```python
from build123d import *

# Parameters (mm, degrees)
F1_DEPTH  = 4
F3_DEPTH  = 7
F5_DEPTH  = 4
F6_R      = 9
F7_DEPTH  = 4
F8_R      = 9
F9_DEPTH  = 4
F10_R     = 2.5
F11_DEPTH = 1.5
F12_R     = 93.772443
F13_DEPTH = 12.5
F14_R     = 1.5
F15_DEPTH = 11.001
F16_R     = 1.5
F17_DEPTH = 15.001
F18_R     = 2.5
F19_DEPTH = 1.5
F21_DEPTH = 11.001


with BuildPart() as f1:
    # F0 (on Right) → F1 (new body)
    with BuildSketch(Plane.YZ):
        with BuildLine():
            ThreePointArc((37.834946, 8.735705), (19.737718, 6.302024), (1.543294, 7.849729))
            ThreePointArc((1.543294, 7.849729), (-8, 0), (1.543294, -7.849729))
            ThreePointArc((1.543294, -7.849729), (19.737718, -6.302024), (37.834946, -8.735705))
            ThreePointArc((37.834946, -8.735705), (49, 0), (37.834946, 8.735705))
        make_face()
    extrude(amount=F1_DEPTH)

    # F2 (on face) → F3 (join)
    with BuildSketch(Plane.YZ.offset(4)):
        with BuildLine():
            ThreePointArc((13.623219, -6.376131), (25.815239, -6.671862), (37.834946, -8.735705))
            ThreePointArc((37.834946, -8.735705), (49, 0), (37.834946, 8.735705))
            ThreePointArc((37.834946, 8.735705), (19.737718, 6.302024), (1.543294, 7.849729))
            ThreePointArc((1.543294, 7.849729), (0.775296, 7.962344), (0, 8))
            Line((0, 8), (0, 6))
            ThreePointArc((0, 6), (2.468627, 5.468627), (4.5, 3.968627))
            Line((4.5, 3.968627), (13.623219, -6.376131))
        make_face()
    extrude(amount=F3_DEPTH)

    # F4 (on face) → F5 (join)
    with BuildSketch(Plane.YZ.offset(11)):
        with BuildLine():
            ThreePointArc((37.834946, 8.735705), (19.737718, 6.302024), (1.543294, 7.849729))
            ThreePointArc((1.543294, 7.849729), (0.775296, 7.962344), (0, 8))
            ThreePointArc((0, 8), (-7.962344, -0.775296), (1.543294, -7.849729))
            ThreePointArc((1.543294, -7.849729), (7.556447, -6.893156), (13.623219, -6.376131))
            ThreePointArc((13.623219, -6.376131), (25.815239, -6.671862), (37.834946, -8.735705))
            ThreePointArc((37.834946, -8.735705), (49, 0), (37.834946, 8.735705))
        make_face()
    extrude(amount=F5_DEPTH)

    # F6 (on face) → F7 (cut)
    with BuildSketch(Plane.YZ.offset(15)):
        with Locations((40, 0)):
            Circle(F6_R)
    extrude(amount=-F7_DEPTH, mode=Mode.SUBTRACT)

    # F8 (on face) → F9 (cut)
    with BuildSketch(Plane(origin=(0, 0, 0), x_dir=(0, -1, 0), z_dir=(-1, 0, 0))):
        with Locations((-40, 0)):
            Circle(F8_R)
    extrude(amount=-F9_DEPTH, mode=Mode.SUBTRACT)

    # F10 (on face) → F11 (cut)
    with BuildSketch(Plane(origin=(0, 0, 0), x_dir=(0, -1, 0), z_dir=(-1, 0, 0))):
        Circle(F10_R)
    extrude(amount=-F11_DEPTH, mode=Mode.SUBTRACT)

    # F12 (on Top) → F13 (cut, symmetric)
    with BuildSketch(Plane.XY):
        with Locations((-92, 19.68912)):
            Circle(F12_R)
        with Locations((107, 19.68912)):
            Circle(F12_R)
    extrude(amount=F13_DEPTH, both=True, mode=Mode.SUBTRACT)

    # F14 (on face) → F15 (cut, through all)
    with BuildSketch(Plane.YZ.offset(11)):
        with Locations((40, 0)):
            Circle(F14_R)
    extrude(amount=-F15_DEPTH, mode=Mode.SUBTRACT)

    # F16 (on face) → F17 (cut, through all)
    with BuildSketch(Plane.YZ.offset(15)):
        Circle(F16_R)
    extrude(amount=-F17_DEPTH, mode=Mode.SUBTRACT)

    # F18 (on face) → F19 (cut)
    with BuildSketch(Plane.YZ.offset(15)):
        Circle(F18_R)
    extrude(amount=-F19_DEPTH, mode=Mode.SUBTRACT)

    # F20 (on face) → F21 (cut, through all)
    with BuildSketch(Plane.YZ.offset(11)):
        with BuildLine():
            ThreePointArc((40, 7), (46.67877, 2.096194), (44, -5.744563))
            Line((44, -5.744563), (39.357692, -8.977051))
            ThreePointArc((39.357692, -8.977051), (48.994261, -0.321359), (40, 9))
            Line((40, 9), (40, 7))
        make_face()
    extrude(amount=-F21_DEPTH, mode=Mode.SUBTRACT)


solid = f1.part
```
Work out the finished part from the listing and answer in its coordinate system (mm). A direction names the side the tool comes from. Give positions to 0.01 mm unless a question says otherwise; leave off trailing zeros. Loops run counter-clockwise (first coordinate to the right, second up) from the corner with the lowest first, then second, coordinate; pieces in that order, holes last. Notation, with made-up numbers: (55, 33.25) -> (65, 33.25) arc R16 cw to (65, 54.25) -> close; hole circle Ø7 at (-27.75, 77.5). An arc over 180 degrees is marked (long way). One line per question, with ' | ' between items. Start each with the question number.
1) Section A-A, the plane x = 10.5 is taken. Determine the outline of the cut face in (y, z).
2) Section B-B, the plane z = 0 is taken. State how many separate pieces and enclosed holes the cut face has, then the cut area to 3 significant figures.
3) Determine the mould class of faces 1 (the face through (11, 0, -2)), 2 (the face through (9.42, 0.79, 7.96)), 3 (the face through (7.55, 38.5, 0.07)), 4 (the face through (7.5, 2.4, 5.5)) for opening direction Z: +Z half, -Z half, draft (parallel to the pull), parting line (faces both ways), or undercut.
4) Section C-C, the plane y = 24 is taken. Determine the outline of the cut face in (x, z).
5) For faces 5 (the face through (11, 37, 0)), 6 (the face through (0.74, -2.385, 0.751)), 7 (the face through (7.451, 8.998, -1.131)), 8 (the face through (8, 40, 8)), 9 (the face through (4, 37, 0)), determine the directions among +Z, -Z, +X, -X, +Y, -Y from which every point of the face is accessible in a straight line to the end or side of a thin tool.
6) Section D-D, the plane z = -4 is taken. Determine the outline of the cut face in (x, y), then the cut area to 3 significant figures.
7) Each of these flat-tipped pins is pushed along its axis until it touches: pin 1 (5 mm diameter, centred on y = 40, z = 0, fed in from -X); pin 2 (3 mm diameter, centred on x = 5.5, y = 32.5, fed in from -Z); pin 3 (1 mm diameter, centred on x = 12, z = 4.5, fed in from -Y). Where does it stop, or does it pass through?
8) Straight lines are drawn through the part: L1, parallel to X at y = 0, z = -3.75; L2, parallel to Z at x = 2.75, y = 0; L3, parallel to X at y = 11, z = -4.75. For each, find the intervals that lie inside material, in ascending order.
Resolved:
1) outline: (0, 6) arc R6 cw to (4.5, 3.97) -> (13.62, -6.38) arc R83.72 cw to (37.83, -8.74) arc R9 ccw to (39.36, -8.98) -> (44, -5.74) arc R7 ccw to (40, 7) -> (40, 9) arc R9 ccw to (37.83, 8.74) arc R83.72 cw to (1.54, 7.85) arc R8 ccw to (0, 8) -> close; hole circle Ø3 at (40, 0)
2) separate pieces: 4 | enclosed holes: 0 | area: 456 mm2
3) face 1: draft | face 2: +Z half | face 3: undercut | face 4: -Z half
4) outline: (1.67, -6.51) -> (13.33, -6.51) -> (13.33, 6.51) -> (1.67, 6.51) -> close
5) face 5: +X, +Y | face 6: -X | face 7: -Z, -Y | face 8: +Z, +X, -X, +Y | face 9: -X, +Y
6) outline: (0, -6.93) -> (4, -6.93) -> (4, 11.53) -> (11, 11.53) -> (11, -6.93) -> (15, -6.93) -> (15, 1.54) arc R93.77 cw to (14.03, 31.94) -> (11, 31.94) -> (11, 45.74) -> (4, 45.74) -> (4, 31.94) -> (0.97, 31.94) arc R93.77 cw to (0, 1.54) -> close | area: 471 mm2
7) pin 1: x = 4 | pin 2: z = -7.88 | pin 3: y = -6.93
8) L1: 0 to 4, 11 to 15 | L2: -8 to -1.5, 1.5 to 8 | L3: 1.37 to 4, 11 to 13.63
